Geometry: see drawing. Coordinates: mm, zero at the bounding-box minimum. Round coordinates to 2 decimals unless told otherwise and drop trailing zeros. Order: outer loops, then holes, each group sorted by start corner. A loop starts at its lowest first (then second) coordinate and runs counter-clockwise, first axis right, second up. Notation, with made-up numbers: (-23, -4) -> (30, -4) arc R14 ccw to (30, 12) -> close; hole circle Ø1 at (33, -9.75). An arc over 180 degrees is marked (long way). Answer as CSV lines item,"result". Start each with the question number.
(1) Section query A-A (z = 1.15). Output: boundary loops of the cut face in (x, y), plus the area to 3 significant figures.
(2) Section query C-C (y = 38.5). Output: boundary loops of the cut face in (x, z).
(3) Line query: line 1 along Y through (x, z) = (122, 4.55); line 2 along Y through (x, z) = (122.5, 0.55); line 3 along X through (y, z) = (131.5, 2.85). Output: solid intervals per line, ascending. Write a range as from..to.
(4) Section query D-D (x = 25.5). Output: boundary loops of the cut face in (y, z), plus the area to 3 significant figures.
(5) Contact query for flat-ended pins moving along their axis: P1, Ø3, axis at x = 105, z = 4, coming from the -Y side; P2, Ø9, axis at x = 123.094, y = 90, coming from the -Z side; P3, Ø3, axis at y = 86.5, z = 1, coming from the -X side. Output: stop coordinate, or through.
(6) Section query B-B (y = 90). Output: boundary loops of the cut face in (x, z), plus the area to 3 significant figures.
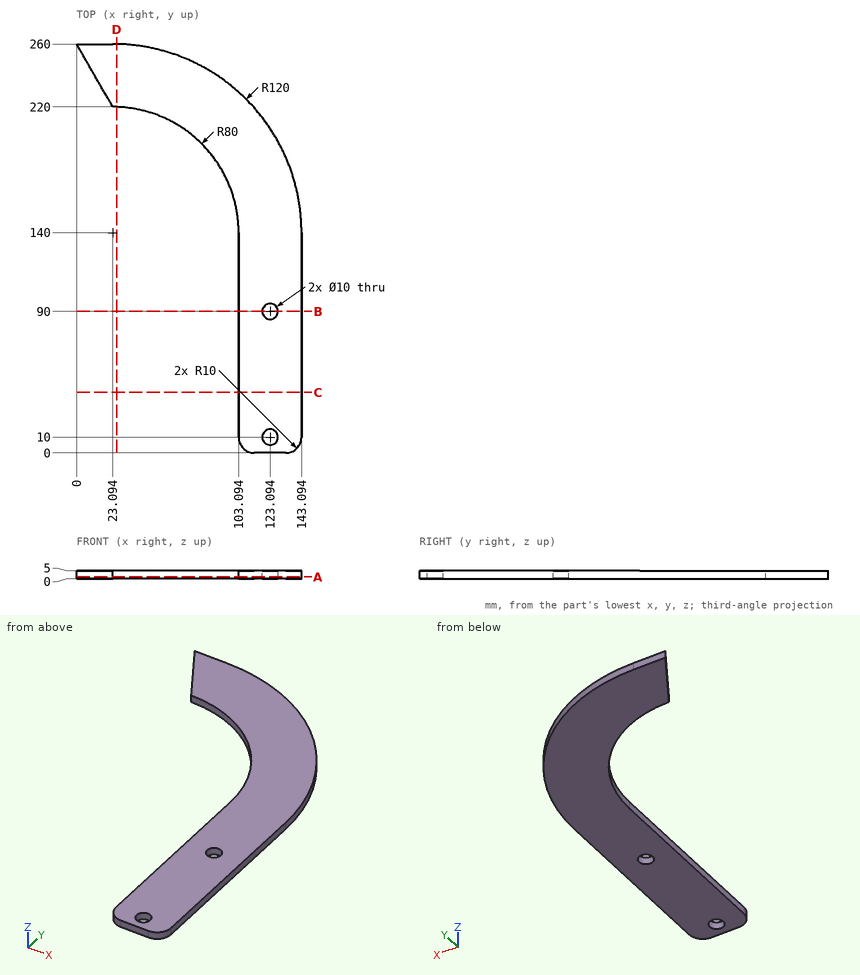
Answer block:
1,outline,"(0, 260) -> (23.09, 220) arc R80 cw to (103.09, 140) -> (103.09, 10) arc R10 ccw to (113.09, 0) -> (133.09, 0) arc R10 ccw to (143.09, 10) -> (143.09, 140) arc R120 ccw to (23.09, 260) -> close; hole circle Ø10 at (123.09, 10); hole circle Ø10 at (123.09, 90)"
1,area,"12,100 mm2"
2,outline,"(103.09, 0) -> (143.09, 0) -> (143.09, 5) -> (103.09, 5) -> close"
3,line 1,"0..5.12, 14.88..85.12, 94.88..207.95"
3,line 2,"0..5.04, 14.96..85.04, 94.96..207.22"
3,line 3,"103.09..143.09"
4,outline,"(219.96, 0) -> (259.98, 0) -> (259.98, 5) -> (219.96, 5) -> close"
4,area,"200 mm2"
5,P1,"y = 2.48"
5,P2,"through"
5,P3,"x = 103.09"
6,outline,"(103.09, 0) -> (118.09, 0) -> (118.09, 5) -> (103.09, 5) -> close; (128.09, 0) -> (143.09, 0) -> (143.09, 5) -> (128.09, 5) -> close"
6,area,"150 mm2"
